Build history of the part. All positions in model axes, mm. A direction names the side the tool comes from. Round coordinates to 2 decimals unless told otherwise and drop trailing zeros. Order: outer loops, then holes, each group sorted by start corner. A loop starts at its lowest first (then second) coordinate and runs counter-clockwise, first axis right, second up. Notation, with made-up numbers: (46.5, -9) -> (51.5, -9) arc R19 ccw to (51.5, 15) -> close; hole circle Ø8 at (-15.5, -11.5). An arc over 180 degrees is marked (long way). Answer as CSV lines item,"result". Start each with the question number.
```python
from build123d import *

# Parameters (mm, degrees)
SKETCH001_R        = 1.7
POCKET_DEPTH       = 455.315212
POLARPATTERN_COUNT = 3


with BuildPart() as part:
    # Sketch → Revolution (revolve)
    with BuildSketch(Plane.XZ):
        Polygon((55, 13), (55, 27.5), (75, 27.5), (75, 0), (57.568888, 0), (57.568888, 6.5), (49, 12.5), (49, 13), align=None)
    revolve(axis=Axis((0, 0, 0), (0, 0, 1)))

    # Sketch001 (on Face2 of Revolution) → Pocket (cut, through all)
    with BuildSketch(Plane(origin=(0, 0, 27.5), x_dir=(-1, 0, 0), z_dir=(0, 0, 1))):
        with Locations((-67.5, 0)):
            Circle(SKETCH001_R)
    pocket = extrude(amount=-POCKET_DEPTH, mode=Mode.SUBTRACT)

    # PolarPattern: Pocket ×3 about axis
    polarpattern_axis = Axis((0, 0, 27.5), (0, 0, 1))
    for i in range(1, POLARPATTERN_COUNT):
        add(pocket.rotate(polarpattern_axis, i * 360 / POLARPATTERN_COUNT), mode=Mode.SUBTRACT)


solid = part.part
```
Q1. Slice it at D-D, the plane y = -65.5. Write the cut outline in (x, z).
Q2. Which spindle directions (+Z, -Z, +X, -X, +Y, -Y) get a long thin tool onto all of the face, cutting with end or side? Do faces 4 (the face through (-11.923, -53.692, 20.352)), 5 (the face through (-34.66, 57.02, 13.94)), 6 (the face through (-7.49, 57.08, 3.3)). Say none if no direction does.
Q3. Flat gauge pins, fed straight in: pin 1 Ø8 at (x, y) = (35, 36) entering from +Z; pin 2 Ø12 at (x, y) = (34.5, 42) entering from +Z; pin 3 Ø4 at (y, z) = (30, 14) entering from -X; pin 4 Ø2 at (x, y) = (67.5, 0) entering from +Z. Where does each tip first touch, or does it go through?
Q4. Slice it at B-B, the plane z = 3.5. Write the cut outline in (x, y).
Q5. Probe L1, parallel to Y at x = 0, z = 23; L2, parallel to Y at x = -33.75, z = 10.75; L3, parallel to Y at x = 0, z = 1.75. List the from-to ranges inside material, lowest first.
Q6. Two-plate mould, pull along X, no slides. Class faces 1 (the face through (-9.764, 74.362, 13.558)), 2 (the face through (22.57, 50.35, 27.5)), 3 (the face through (-6.433, 48.996, 12.209)): +X half, -X half, draft (parallel to the pull), parting line (faces both ways), or undercut.
Q7. Slice it at A-A, the plane x = 0. Write the cut outline in (y, z).
Q8. Slice it at C-C, the plane x = 60. Write the cut outline in (y, z), plus the area to 4 significant figures.
Solutions:
1,outline,"(-36.53, 0) -> (36.53, 0) -> (36.53, 27.5) -> (-36.53, 27.5) -> close"
2,face 4,"+Z"
2,face 5,"+Z, -Z"
2,face 6,"-Z"
3,pin 1,"stops at z = 13"
3,pin 2,"stops at z = 27.5"
3,pin 3,"stops at x = -69.58"
3,pin 4,"passes through"
4,outline,"circle Ø150 at (0, 0); hole circle Ø115.14 at (0, 0); hole circle Ø3.4 at (-33.75, -58.46); hole circle Ø3.4 at (-33.75, 58.46); hole circle Ø3.4 at (67.5, 0)"
5,L1,"y = -75 to -55, 55 to 75"
5,L2,"y = -66.98 to -60.16, -56.76 to -38.9, 38.9 to 56.76, 60.16 to 66.98"
5,L3,"y = -75 to -57.57, 57.57 to 75"
6,face 1,"parting line"
6,face 2,"draft"
6,face 3,"undercut"
7,outline,"(-75, 0) -> (-57.57, 0) -> (-57.57, 6.5) -> (-49, 12.5) -> (-49, 13) -> (-55, 13) -> (-55, 27.5) -> (-75, 27.5) -> close; (49, 12.5) -> (57.57, 6.5) -> (57.57, 0) -> (75, 0) -> (75, 27.5) -> (55, 27.5) -> (55, 13) -> (49, 13) -> close"
8,outline,"(-45, 0) -> (45, 0) -> (45, 27.5) -> (-45, 27.5) -> close"
8,area,"2,475 mm2"
